from build123d import *

# Parameters (mm, degrees)
SKETCH1_W                        = 203.2
SKETCH1_H                        = 304.8
BOSS_EXTRUDE1_DEPTH              = 3.175
F_1_4_CLEARANCE_HOLE1_AT_2_COUNT = 2
F_1_4_CLEARANCE_HOLE1_AT_2_PITCH = 165.1
F_1_4_CLEARANCE_HOLE1_AT_3_COUNT = 2
F_1_4_CLEARANCE_HOLE1_AT_3_PITCH = 313.666861495
F_1_4_CLEARANCE_HOLE1_AT_4_COUNT = 2
F_1_4_CLEARANCE_HOLE1_AT_4_PITCH = 266.7
CHAMFER1_SIZE                    = 0.508


with BuildPart() as part:
    # Sketch1 → Boss-Extrude1 (new body, symmetric)
    with BuildSketch(Plane(origin=(0, 0, 0), x_dir=(1, 0, 0), z_dir=(0, 1, 0))):
        Rectangle(SKETCH1_W, SKETCH1_H)
    extrude(amount=BOSS_EXTRUDE1_DEPTH, both=True)

    # Sketch4 → 1_4 Clearance Hole1 (revolve, cut)
    with BuildSketch(Plane(origin=(-82.55, 3.175, -133.35), x_dir=(0, 0, 1), z_dir=(1, 0, 0))):
        Polygon((0, 0), (0, 6.35), (3.82524, 6.35), (3.57124, 6.096), (3.57124, 0.254), (3.82524, 0), align=None)
    f_1_4_clearance_hole1 = revolve(axis=Axis((-82.55, 9.525, -133.35), (0, -1, 0)), mode=Mode.SUBTRACT)

    # 1_4 Clearance Hole1 at 2: 1_4 Clearance Hole1 ×2
    with Locations(*[(i * F_1_4_CLEARANCE_HOLE1_AT_2_PITCH, 0, 0) for i in range(1, F_1_4_CLEARANCE_HOLE1_AT_2_COUNT)]):
        add(f_1_4_clearance_hole1, mode=Mode.SUBTRACT)

    # 1_4 Clearance Hole1 at 3: 1_4 Clearance Hole1 ×2
    with Locations(*[Vector(0.526354615, 0, 0.850265147) * (i * F_1_4_CLEARANCE_HOLE1_AT_3_PITCH) for i in range(1, F_1_4_CLEARANCE_HOLE1_AT_3_COUNT)]):
        add(f_1_4_clearance_hole1, mode=Mode.SUBTRACT)

    # 1_4 Clearance Hole1 at 4: 1_4 Clearance Hole1 ×2
    with Locations(*[(0, 0, i * F_1_4_CLEARANCE_HOLE1_AT_4_PITCH) for i in range(1, F_1_4_CLEARANCE_HOLE1_AT_4_COUNT)]):
        add(f_1_4_clearance_hole1, mode=Mode.SUBTRACT)

    # Chamfer1
    chamfer1_edges = [part.edges().sort_by_distance(p)[0] for p in [
        (-101.6, 3.175, 0),
        (0, 3.175, 152.4),
        (101.6, 3.175, 0),
        (0, -3.175, 152.4),
        (-101.6, -3.175, 0),
        (0, -3.175, -152.4),
        (101.6, -3.175, 0),
        (101.6, 0, 152.4),
        (-101.6, 0, 152.4),
        (-101.6, 0, -152.4),
        (101.6, 0, -152.4),
        (0, 3.175, -152.4),
    ]]
    chamfer(chamfer1_edges, length=CHAMFER1_SIZE)


solid = part.part
Read the model definition and answer for the solid it produces. Units are mm, in the model's axes. Coordinates: 2 decimals unless noted, no trailing zeros. Loops run counter-clockwise (first coordinate to the right, second up) from the corner with the lowest first, then second, coordinate; pieces in that order, holes last. Notation, with made-up numbers: (-35.75, 13) - (0.25, 13) arc R26 cw to (0.25, 45) - close; hole circle Ø11 at (-10, -3.5). An arc over 180 degrees is marked (long way). Answer in a Markdown table with one row per item.
Q1. Find section A-A on x = -82.55. Write down the section's boundary in (y, z) (3 decimals), plus the area to 3 significant figures.
Here are the results:
| item | result |
|---|---|
| outline | (-3.175, -151.892) - (-2.667, -152.4) - (2.667, -152.4) - (3.175, -151.892) - (3.175, -137.175) - (2.921, -136.921) - (-2.921, -136.921) - (-3.175, -137.175) - close; (-3.175, -129.525) - (-2.921, -129.779) - (2.921, -129.779) - (3.175, -129.525) - (3.175, 129.525) - (2.921, 129.779) - (-2.921, 129.779) - (-3.175, 129.525) - close; (-3.175, 137.175) - (-2.921, 136.921) - (2.921, 136.921) - (3.175, 137.175) - (3.175, 151.892) - (2.667, 152.4) - (-2.667, 152.4) - (-3.175, 151.892) - close |
| area | 1,840 mm^2 |
Q2. Straight lines are drawn through the part: line 1 along Z through (x, y) = (-82.55, 0.1); line 2 along X through (y, z) = (0.75, -133.35); line 3 along X through (y, z) = (2.75, -50). For each, find the intervals that lie inside material, in ascending order. Write a range as [from, to].
Here are the results:
| item | result |
|---|---|
| line 1 | z = [-152.4, -136.92], [-129.78, 129.78], [136.92, 152.4] |
| line 2 | x = [-101.6, -86.12], [-78.98, 78.98], [86.12, 101.6] |
| line 3 | x = [-101.52, 101.52] |
Q3. The mould has two halves that part along Z. Classify faces 1 (the flat face through (-1, 3.175, -2)), 2 (the cylindrical face through (-86.09, 0.04, 132.89)): pulls with the +Z half, pulls with the -Z half, needs draft (parallel to the pull), parting line crosses it, or undercut.
Here are the results:
| item | result |
|---|---|
| face 1 | needs draft |
| face 2 | undercut |
Q4. Find section B-B on z = 133.35. Write down the section's boundary in (x, y) (3 decimals).
Here are the results:
| item | result |
|---|---|
| outline | (-101.6, -2.667) - (-101.092, -3.175) - (-86.375, -3.175) - (-86.121, -2.921) - (-86.121, 2.921) - (-86.375, 3.175) - (-101.092, 3.175) - (-101.6, 2.667) - close; (-78.979, -2.921) - (-78.725, -3.175) - (78.725, -3.175) - (78.979, -2.921) - (78.979, 2.921) - (78.725, 3.175) - (-78.725, 3.175) - (-78.979, 2.921) - close; (86.121, -2.921) - (86.375, -3.175) - (101.092, -3.175) - (101.6, -2.667) - (101.6, 2.667) - (101.092, 3.175) - (86.375, 3.175) - (86.121, 2.921) - close |
